Verification items for the finished model (mm, model axes). A direction names the side the tool comes from. Coordinates: 2 decimals unless noted, no trailing zeros. Loops run counter-clockwise (first coordinate to the right, second up) from the corner with the lowest first, then second, coordinate; pieces in that order, holes last.
Q1. Material ranges on probe 1 along Y at (x, z) = (32, 1.9); probe 2 along X at (y, z) = (32, 1); probe 3 along Y at (x, z) = (-1, 1.7), recorded low to high.
Q2. Sectioned sample at A-A (y = -16). Enter the section's corners in (x, z).
Q3. Sectioned sample at B-B (x = 33). Enter the section's corners in (y, z).
Q4. Access from +Z, -Z, +X, -X, +Y, -Y to the whole of each face (thin tool, end or side, straight path). Record for faces 1 (the face through (30, 61.243, 1)), 2 (the face through (29, 46.726, 1)), 3 (the face through (29, -32.957, 1)).
Q5. Go/stop test with flat-tipped pins: P1, Ø1, axis at x = 40, z = 1, coming from the +Y side; P2, Ø0.6, axis at y = 21, z = 1, coming from the +X side; P3, Ø3, axis at x = 51.22, y = 50.22, coming from the -Z side. Record where each tip stops, or that it passes through.
Q6. Mould release check, pull along X, two halves, no side actions. Record for faces 4 (the face through (2, 26, 0)), 5 (the face through (29, -22.274, 1)), 6 (the face through (0.123, 15, 1)): +X half, -X half, draft (parallel to the pull), parting line (faces both ways), or undercut.
Q7. Sectioned sample at C-C (z = 0.45). Count the separate pieces of the cut face and the enclosed holes in it, then the cut area to 3 significant figures.
Q8. Sectioned sample at D-D (x = 51). Enter the section's corners in (y, z).
```python
from build123d import *

# Parameters (mm, degrees)
SKETCH1_R           = 1.55
SKETCH1_R_2         = 1.552736715
SKETCH1_W           = 50.2
SKETCH1_H           = 69
BOSS_EXTRUDE1_DEPTH = 2
SKETCH2_R           = 2.09
CUT_EXTRUDE1_DEPTH  = 10


with BuildPart() as part:
    # Sketch1 → Boss-Extrude1 (new body)
    with BuildSketch(Plane.XY):
        with BuildLine():
            Line((54.323201224, 61.242975378), (4.123201224, 61.242975378))
            ThreePointArc((4.123201224, 61.242975378), (-2.705225901, 64.071402503), (0.123201224, 57.242975378))
            Line((0.123201224, 57.242975378), (0.123201224, -28.957024622))
            ThreePointArc((0.123201224, -28.957024622), (-2.705225901, -35.785451747), (4.123201224, -32.957024622))
            Line((4.123201224, -32.957024622), (54.323201224, -32.957024622))
            ThreePointArc((54.323201224, -32.957024622), (61.151628348, -35.785451747), (58.323201224, -28.957024622))
            Line((58.323201224, -28.957024622), (58.323201224, 57.242975378))
            ThreePointArc((58.323201224, 57.242975378), (61.151628348, 64.071402503), (54.323201224, 61.242975378))
        make_face()
        with Locations((7.223201224, 50.222695663)):
            Circle(SKETCH1_R, mode=Mode.SUBTRACT)
        with Locations((51.223201224, 50.222975378)):
            Circle(SKETCH1_R, mode=Mode.SUBTRACT)
        with Locations((7.233060223, -25.857304337)):
            Circle(SKETCH1_R_2, mode=Mode.SUBTRACT)
        with Locations((51.223201224, -25.857024622)):
            Circle(SKETCH1_R, mode=Mode.SUBTRACT)
        with Locations((29.223201224, 12.225914551)):
            Rectangle(SKETCH1_W, SKETCH1_H, mode=Mode.SUBTRACT)
    extrude(amount=BOSS_EXTRUDE1_DEPTH)

    # Sketch2 → Cut-Extrude1 (cut)
    with BuildSketch(Plane.XY.offset(2)):
        with Locations((0.123201224, 61.242975378)):
            Circle(SKETCH2_R)
        with Locations((58.323201224, 61.242975378)):
            Circle(SKETCH2_R)
        with Locations((0.123201224, -32.957024622)):
            Circle(SKETCH2_R)
        with Locations((58.323201224, -32.957024622)):
            Circle(SKETCH2_R)
    extrude(amount=-CUT_EXTRUDE1_DEPTH, mode=Mode.SUBTRACT)


solid = part.part
```
Geometry check:
1. probe 1: y = -32.96 to -22.27, 46.73 to 61.24
1. probe 2: x = 0.12 to 4.12, 54.32 to 58.32
1. probe 3: y = -36.8 to -34.72, -31.19 to -29.12, 57.4 to 59.48, 63.01 to 65.08
2. outline: (0.12, 0) - (4.12, 0) - (4.12, 2) - (0.12, 2) - close; (54.32, 0) - (58.32, 0) - (58.32, 2) - (54.32, 2) - close
3. outline: (-32.96, 0) - (-22.27, 0) - (-22.27, 2) - (-32.96, 2) - close; (46.73, 0) - (61.24, 0) - (61.24, 2) - (46.73, 2) - close
4. face 1: +Z, -Z, +Y
4. face 2: +Z, -Z
4. face 3: +Z, -Z, -Y
5. P1: stops at y = 61.24
5. P2: stops at x = 58.32
5. P3: passes through
6. face 4: draft
6. face 5: undercut
6. face 6: -X half
7. separate pieces: 1
7. enclosed holes: 9
7. area: 2,080 mm2
8. outline: (-32.96, 0) - (-27.39, 0) - (-27.39, 2) - (-32.96, 2) - close; (-24.32, 0) - (-22.27, 0) - (-22.27, 2) - (-24.32, 2) - close; (46.73, 0) - (48.69, 0) - (48.69, 2) - (46.73, 2) - close; (51.76, 0) - (61.24, 0) - (61.24, 2) - (51.76, 2) - close
